Geometry: final body of the model. Coordinates: model frame, mm. A direction names the side the tool comes from. Round coordinates to 2 decimals unless told otherwise and drop trailing zeros. Loops run counter-clockwise (first coordinate to the right, second up) from the corner with the lowest first, then second, coordinate; pieces in that order, holes last. Notation, with made-up numbers: M 79.5,62 L 104.5,62 A24 cw 104.5,83 Z; hole C -5,17 d6. An arc over 180 degrees is marked long. Answer as a JSON object with one key per item and string values.
```python
from build123d import *

# Parameters (mm, degrees)
SKETCH1_R           = 25.4
BOSS_EXTRUDE2_DEPTH = 33.274
SKETCH2_R           = 22.225
BOSS_EXTRUDE3_DEPTH = 19.05
SKETCH3_R           = 12.7
CUT_EXTRUDE1_DEPTH  = 64.467479673
BOSS_EXTRUDE4_DEPTH = 25.4
FILLET1_R           = 6.35
CUT_EXTRUDE3_DEPTH  = 154.252958066
BOSS_EXTRUDE5_DEPTH = 8.128
FILLET2_R           = 6.35


with BuildPart() as part:
    # Sketch1 → Boss-Extrude2 (new body)
    with BuildSketch(Plane.XY):
        Circle(SKETCH1_R)
    extrude(amount=BOSS_EXTRUDE2_DEPTH)

    # Sketch2 → Boss-Extrude3 (add)
    with BuildSketch(Plane.XY.offset(33.274)):
        with Locations(Location((0, 0, 0), (0, 0, 180))):
            Circle(SKETCH2_R)
    extrude(amount=BOSS_EXTRUDE3_DEPTH)

    # Sketch3 → Cut-Extrude1 (cut, through all)
    with BuildSketch(Plane.XY):
        Circle(SKETCH3_R)
    extrude(amount=CUT_EXTRUDE1_DEPTH, mode=Mode.SUBTRACT)

    # Sketch6 → Boss-Extrude4 (add)
    with BuildSketch(Plane.XY.offset(2.54)):
        with BuildLine():
            Line((21.997045256, 12.7), (100.803124952, 12.7))
            ThreePointArc((100.803124952, 12.7), (96.298711326, 32.390094118), (87.988181024, 50.8))
            ThreePointArc((87.988181024, 50.8), (92.636703653, 68.148522628), (109.985226281, 63.5))
            ThreePointArc((109.985226281, 63.5), (125.578613792, 18.9476056), (123.824497467, -28.222222222))
            ThreePointArc((123.824497467, -28.222222222), (108.619825498, -37.782449747), (99.059597973, -22.577777778))
            ThreePointArc((99.059597973, -22.577777778), (100.053333913, -17.660418251), (100.803124952, -12.7))
            Line((100.803124952, -12.7), (21.997045256, -12.7))
            ThreePointArc((21.997045256, -12.7), (-25.4, 0), (21.997045256, 12.7))
        make_face()
    extrude(amount=BOSS_EXTRUDE4_DEPTH)

    # Fillet1
    fillet1_edges = [part.edges().sort_by_distance(p)[0] for p in [
        (100.803124952, -12.7, 15.24),
        (100.803124952, 12.7, 15.24),
    ]]
    fillet(fillet1_edges, radius=FILLET1_R)

    # Sketch7 → Cut-Extrude3 (cut, through all)
    with BuildSketch(Plane.XY.offset(2.54)):
        with BuildLine():
            Line((41.834095467, -5.588), (72.766466105, -5.588))
            ThreePointArc((72.766466105, -5.588), (78.354466105, 0), (72.766466105, 5.588))
            Line((72.766466105, 5.588), (41.834095467, 5.588))
            ThreePointArc((41.834095467, 5.588), (36.246095467, 0), (41.834095467, -5.588))
        make_face()
        with BuildLine():
            ThreePointArc((117.633272593, -26.811111111), (119.299683103, 18.00022532), (104.485964967, 60.325))
            ThreePointArc((104.485964967, 60.325), (95.811703653, 62.649261314), (93.487442339, 53.975))
            ThreePointArc((93.487442339, 53.975), (106.741821724, 16.10546476), (105.250822847, -23.988888889))
            ThreePointArc((105.250822847, -23.988888889), (110.030936609, -31.591224873), (117.633272593, -26.811111111))
        make_face()
    extrude(amount=CUT_EXTRUDE3_DEPTH, mode=Mode.SUBTRACT)

    # Sketch8 → Boss-Extrude5 (add)
    with BuildSketch(Plane.XY.offset(8.128)):
        with BuildLine():
            Line((21.997045256, 12.7), (93.3255592, 12.7))
            ThreePointArc((93.3255592, 12.7), (98.24424805, 15.033907372), (99.547263147, 20.32))
            ThreePointArc((99.547263147, 20.32), (96.421789325, 32.021844783), (91.925992057, 43.268602754))
            Line((91.925992057, 43.268602754), (0, 25.4))
            ThreePointArc((0, 25.4), (12.7, 21.997045256), (21.997045256, 12.7))
        make_face()
    extrude(amount=BOSS_EXTRUDE5_DEPTH)

    # Fillet2
    # the kernel refuses this fillet: 6.35 mm, written as the material it adds along each edge
    with BuildSketch(Plane(origin=(91.925992057, 43.268602754, 8.128), x_dir=(-0.46401221312407714, 0.8858288017849137, 0), z_dir=(0, 0, 1))) as fillet2_piece_1:
        with BuildLine():
            CenterArc((8.525728186, 6.347859775), FILLET2_R, 163.353687105, 108.13393528)
            Line((2.441848203, 8.166899178), (1.833460205, 8.348803118))
            Line((1.833460205, 8.348803118), (-0.608387998, 0.18190394))
            Line((-0.608387998, 0.18190394), (-0.027038803, -0.634424072))
            ThreePointArc((-0.027038803, -0.634424072), (8.524799214, -0.640898159), (8.707065713, -0.634785977))
            Line((8.707065713, -0.634785977), (8.690580483, 0))
        make_face()
    extrude(amount=8.128)


solid = part.part
```
1) Line query: probe 1 along Y at (x, z) = (0, 1); probe 2 along Y at (x, z) = (0, 44.75) (3 decimals); probe 3 along X at (y, z) = (-14.5, 22.5) (1 decimal). Output: solid intervals per line, ascending.
Geometry results:
{"probe 1": "-25.4 to -12.7, 12.7 to 25.4", "probe 2": "-22.225 to -12.7, 12.7 to 22.225", "probe 3": "-20.9 to 20.9, 97.8 to 107, 119.8 to 126.2"}
2) Cut plane C-C on y = 57.15. Return the cut outline in (x, z).
Geometry results:
{"outline": "M 86.29,2.54 L 92.64,2.54 L 92.64,27.94 L 86.29,27.94 Z; M 106.26,2.54 L 113.41,2.54 L 113.41,27.94 L 106.26,27.94 Z"}
3) First-contact query: pin 1 (20.5 mm diameter, centred on x = 0, y = 0, fed in from +Z); pin 2 (6 mm diameter, centred on x = 58, z = 21.5, fed in from -Y); pin 3 (8 mm diameter, centred on y = 12, z = 10, fed in from -X). Flat tips, straight axial feed; report the tip coordinate or a pass-through.
Geometry results:
{"pin 1": "z = 27.94", "pin 2": "y = -12.7", "pin 3": "x = -24.11"}
4) Cut plane A-A on y = 0. Return the cut outline in (x, z) (3 decimals).
Geometry results:
{"outline": "M -25.4,0 L -12.7,0 L -12.7,2.54 L 12.7,2.54 L 12.7,0 L 25.4,0 L 25.4,2.54 L 36.246,2.54 L 36.246,27.94 L 25.4,27.94 L 25.4,33.274 L 22.225,33.274 L 22.225,52.324 L 12.7,52.324 L 12.7,27.94 L -12.7,27.94 L -12.7,52.324 L -22.225,52.324 L -22.225,33.274 L -25.4,33.274 Z; M 78.354,2.54 L 107.95,2.54 L 107.95,27.94 L 78.354,27.94 Z; M 120.65,2.54 L 127,2.54 L 127,27.94 L 120.65,27.94 Z"}
5) Cut plane D-D on x = 6.5. Return the cut outline in (y, z).
Geometry results:
{"outline": "M -24.55,0 L -10.91,0 L -10.91,2.54 L 10.91,2.54 L 10.91,0 L 24.55,0 L 24.55,8.13 L 26.66,8.13 L 26.66,16.26 L 24.55,16.26 L 24.55,33.27 L 21.25,33.27 L 21.25,52.32 L 10.91,52.32 L 10.91,27.94 L -10.91,27.94 L -10.91,52.32 L -21.25,52.32 L -21.25,33.27 L -24.55,33.27 Z"}
6) Cut plane B-B on z = 48. Return the cut outline in (x, y) (3 decimals).
Geometry results:
{"outline": "C 0,0 d44.45; hole C 0,0 d25.4"}
7) Pull-direction query (X, two-part tool) for faces 1 (the face through (-10, 10, 52.324)), 2 (the face through (98.19, 14.97, 22.18)), 3 (the face through (0, 0, 2.54)), 4 (the face through (88.07, 45.12, 12.14)); classes: +X half, -X half, draft (parallel to the pull), parting line (faces both ways), or undercut.
Geometry results:
{"face 1": "draft", "face 2": "undercut", "face 3": "undercut", "face 4": "-X half"}
8) Set-up query: faces 5 (the face through (16.4, -15, 42.7)), 6 (the face through (106.656, 16.664, 15.062)), 7 (the face through (58, -12.7, 15)), 8 (the face through (61, 26, 8.128)), 9 (the face through (42.364, 33.635, 12.135)). Return all of +Z, -Z, +X, -X, +Y, -Y with unobstructed straight access to the full face (end or side cutting, diameter ignored); none if empty.
Geometry results:
{"face 5": "+Z", "face 6": "+Z, -Z", "face 7": "+Z, -Z, -Y", "face 8": "-Z", "face 9": "+Z, -Z, -X, +Y"}
